from build123d import *

# Parameters (mm, degrees)
ESQUISSE1_R        = 19
BOSS_EXTRU_2_DEPTH = 3


with BuildPart() as part:
    # Esquisse1 → Boss.-Extru.2 (new body)
    with BuildSketch(Plane.XY):
        Circle(ESQUISSE1_R)
        with BuildLine():
            ThreePointArc((2.745524809, 13.728149676), (-0.608438359, 17.239266306), (-3.706523595, 13.500432691))
            ThreePointArc((-3.706523595, 13.500432691), (-12.363713879, 6.567996584), (-13.261688771, -4.486380606))
            ThreePointArc((-13.261688771, -4.486380606), (-14.625423384, -9.146556229), (-9.838455875, -9.960159939))
            ThreePointArc((-9.838455875, -9.960159939), (0.493805045, -13.991288596), (10.516163961, -9.24176907))
            ThreePointArc((10.516163961, -9.24176907), (15.233861743, -8.092710077), (13.54497947, -3.540272752))
            ThreePointArc((13.54497947, -3.540272752), (11.869908833, 7.423292012), (2.745524809, 13.728149676))
        make_face(mode=Mode.SUBTRACT)
    extrude(amount=BOSS_EXTRU_2_DEPTH)


solid = part.part
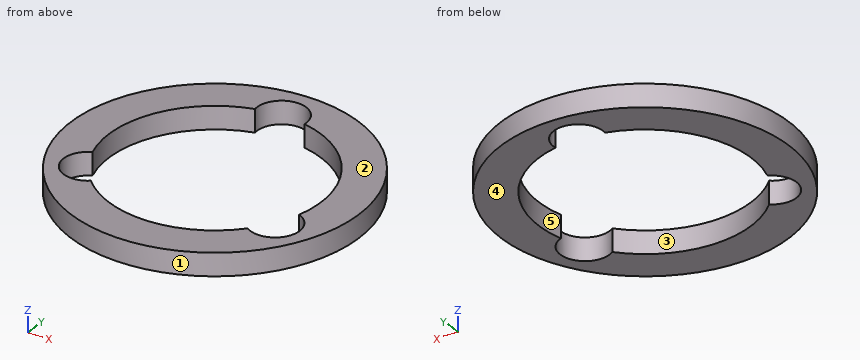
Part model, mm, in its own coordinate system. Face numbers are marked on the shaded views. A direction names the side the tool comes from. Round coordinates to 2 decimals unless told otherwise and drop trailing zeros. Write each loop counter-clockwise with the first axis right and the second up, starting at its lowest first coordinate (ties: lowest second). Pieces come first, ordered by that corner, then holes. Notation, with made-up numbers: M 39,70 L 79,70 A28 cw 79,88 Z; hole C -16,-36 d1. An arc over 180 degrees is marked long. Return JSON: item names as keys, results as strings. Group by question number.
(1) Saw through at B-B on x = 0. Write the cut outline in (y, z), then the cut area to 3 significant figures.
(2) Drill centre lines: probe 1 along X at (y, z) = (-2, 2.7); probe 2 along X at (y, z) = (12.5, 2.55); probe 3 along Y at (x, z) = (2.5, 2.15). Where is each one in solid material? Low to high.
(3) Two-plate mould, pull along X, no slides. Class the marked faces 1, 2 and 3: +X half, -X half, draft (parallel to the pull), parting line (faces both ways), or undercut.
(4) Which spindle directions (+Z, -Z, +X, -X, +Y, -Y) get a long thin tool onto all of the face, cutting with end or side? Do the marked faces 4 and 5. Say none if no direction does.
(5) Saw through at A-A on y = 0. Write the cut outline in (x, z), then the cut area to 3 significant figures.
(6) Pin check, flat tips, straight feed: pin 1 Ø1.5 at (x, z) = (-3, 1.5) entering from +Y; pin 2 Ø1.5 at (x, z) = (10.5, 2) entering from -Y; pin 3 Ø1 at (y, z) = (-11.5, 1.5) entering from +X. Stop position of each tip, or through.
(7) Saw through at C-C on z = 2.55. Write the cut outline in (x, y).
Returned:
{
 "1": {"outline": "M -19,0 L -14,0 L -14,3 L -19,3 Z; M 17.2,0 L 19,0 L 19,3 L 17.2,3 Z", "area": "20.4 mm²"},
 "2": {"probe 1": "-18.89 to -13.86, 13.86 to 18.89", "probe 2": "-14.31 to -6.3, 6.3 to 14.31", "probe 3": "-18.83 to -13.77, 15.26 to 18.83"},
 "3": {"face 1": "parting line", "face 2": "draft", "face 3": "undercut"},
 "4": {"face 4": "-Z, +X, -X, +Y, -Y", "face 5": "+Z, -Z"},
 "5": {"outline": "M -19,0 L -14,0 L -14,3 L -19,3 Z; M 14,0 L 19,0 L 19,3 L 14,3 Z", "area": "30.0 mm²"},
 "6": {"pin 1": "y = 18.87", "pin 2": "y = -16.31", "pin 3": "x = 15.49"},
 "7": {"outline": "C 0,0 d38; hole M -13.26,-4.49 A3.25 ccw long -9.84,-9.96 A14 ccw 10.52,-9.24 A3.25 ccw long 13.54,-3.54 A14 ccw 2.75,13.73 A3.25 ccw long -3.71,13.5 A14 ccw Z"}
}
